Geometry: final body of the model. Coordinates: model frame, mm. Give positions to 0.01 mm unless a question says otherwise; leave off trailing zeros. Order: outer loops, then holes, each group sorted by start corner. A loop starts at its lowest first (then second) coordinate and runs counter-clockwise, first axis right, second up. Notation, with made-up numbers: M -14,-24.75 L 8,-24.75 A17 ccw 8,-15.75 Z; hole C 80,24.5 d4. An arc over 180 degrees is marked long. Use CSV: the item, a comma, the result in double quotes.
```python
from build123d import *

# Parameters (mm, degrees)
SKETCH1_W            = 15.24
SKETCH1_H            = 26.9875
SKETCH5_R            = 14.25575
SEAL_SEAT_DEPTH      = 54.838489136
M6_CLEARANCE_HOLE1_D = 6.6
CIRPATTERN1_COUNT    = 4


with BuildPart() as part:
    # Sketch1 → Main_body (revolve)
    with BuildSketch(Plane(origin=(0, 0, 0), x_dir=(0, 0, -1), z_dir=(1, 0, 0)), mode=Mode.PRIVATE) as main_body_sk:
        with Locations((-127.089000076, -23.01875)):
            Rectangle(SKETCH1_W, SKETCH1_H)
        with Locations((-127.089000076, 23.01875)):
            Rectangle(SKETCH1_W, SKETCH1_H)
    revolve(main_body_sk.sketch.rotate(Axis((0, 0, 1000), (0, 0, -1)), 270), axis=Axis((0, 0, 1000), (0, 0, -1)))

    # Sketch5 → seal_seat (cut, through all)
    with BuildSketch(Plane.XY.offset(134.709000076)):
        Circle(SKETCH5_R)
    extrude(amount=-SEAL_SEAT_DEPTH, mode=Mode.SUBTRACT)

    # M6 Clearance Hole1 (through all)
    with Locations(Plane.XY.offset(134.709000076)):
        with Locations((0, 31.75)):
            m6_clearance_hole1 = Hole(M6_CLEARANCE_HOLE1_D / 2)

    # CirPattern1: M6 Clearance Hole1 ×4 about axis
    cirpattern1_axis = Axis((0, 0, 0), (0, 0, 1))
    for i in range(1, CIRPATTERN1_COUNT):
        add(m6_clearance_hole1.rotate(cirpattern1_axis, i * 360 / CIRPATTERN1_COUNT), mode=Mode.SUBTRACT)


solid = part.part
```
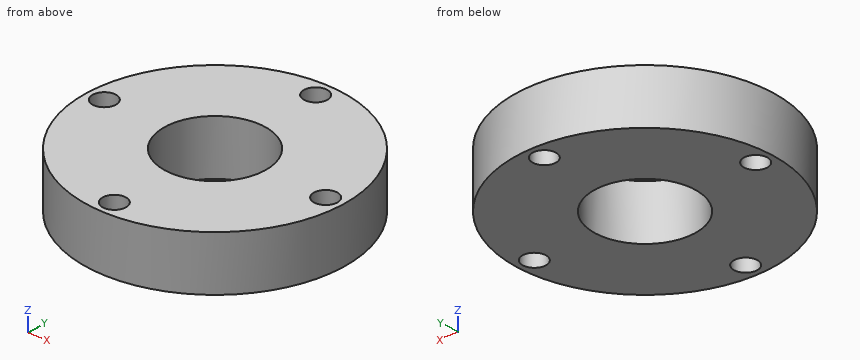
1. Section A-A, the plane y = 0. Return the cut outline in (x, z).
Answer:
outline,"M -36.51,119.47 L -35.05,119.47 L -35.05,134.71 L -36.51,134.71 Z; M -28.45,119.47 L -14.26,119.47 L -14.26,134.71 L -28.45,134.71 Z; M 14.26,119.47 L 28.45,119.47 L 28.45,134.71 L 14.26,134.71 Z; M 35.05,119.47 L 36.51,119.47 L 36.51,134.71 L 35.05,134.71 Z"
2. Line query: line 1 (Y direction, x = 0, z = 125); line 2 (X direction, y = 2, z = 124.5); line 3 (Y direction, x = -11, z = 132.5). Output: solid intervals per line, ascending.
Answer:
line 1,"-36.51 to -35.05, -28.45 to -14.26, 14.26 to 28.45, 35.05 to 36.51"
line 2,"-36.46 to -34.37, -29.13 to -14.11, 14.11 to 29.13, 34.37 to 36.46"
line 3,"-34.82 to -9.07, 9.07 to 34.82"
3. Pin query (flat end, axial travel): pin 1 Ø1.5 at (x, z) = (-4, 127) entering from -Y; pin 2 Ø4 at (x, z) = (-14, 130.5) entering from -Y; pin 3 Ø8 at (y, z) = (-10.5, 133) entering from +X. Return the tip coordinate at first contact, or that it passes through.
Answer:
pin 1,"y = -36.37"
pin 2,"y = -34.48"
pin 3,"x = 35.93"
4. Section C-C, the plane x = 9.5. Return the cut outline in (y, z), plus the area to 3 significant figures.
Answer:
outline,"M -35.25,119.47 L -10.63,119.47 L -10.63,134.71 L -35.25,134.71 Z; M 10.63,119.47 L 35.25,119.47 L 35.25,134.71 L 10.63,134.71 Z"
area,"751 mm2"
5. Section D-D, the plane z = 129.25. Give the number of separate pieces and of enclosed holes in the cut face, plus the area to 3 significant figures.
Answer:
separate pieces,"1"
enclosed holes,"5"
area,"3,410 mm2"
